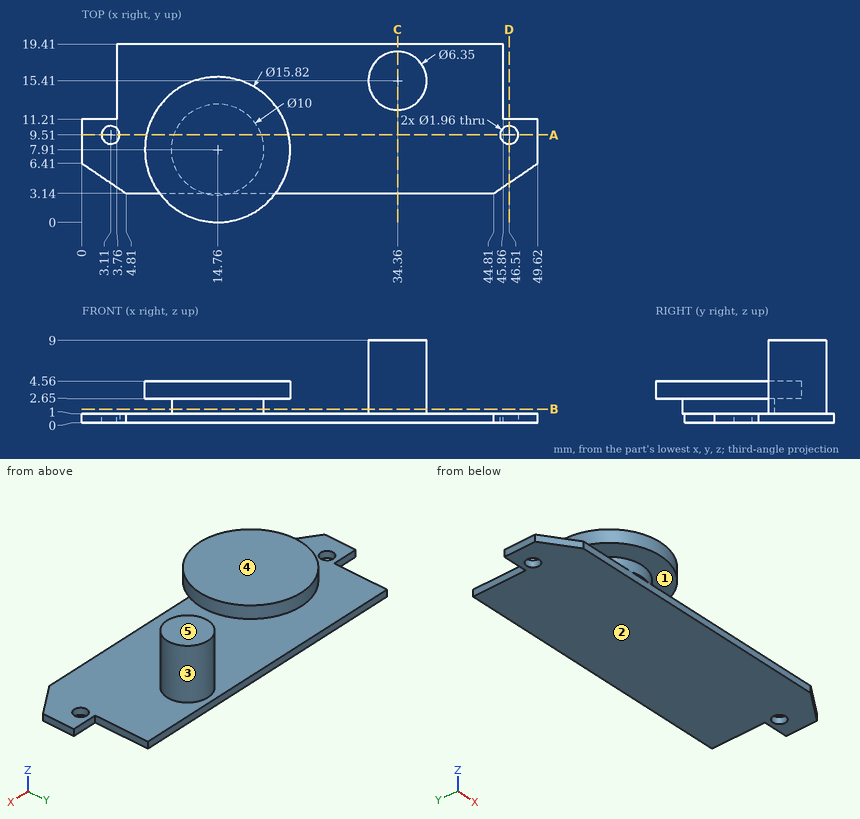
Design review of the part shown in the three views and the two pictorial views. Dimensions are in mm from the part's minimum x, y and z. A direction names the side the tool comes from. Give positions to 0.01 mm unless a question says otherwise; leave off trailing zeros. Write each loop counter-clockwise with the first axis right and the second up, starting at its lowest first coordinate (ties: lowest second). Pieces come first, ordered by that corner, then holes.
(1) Add section D-D (x = 46.51). Give the boundary of the cut face in (y, z).
Checked values:
outline: (4.3, 0) - (8.53, 0) - (8.53, 1) - (4.3, 1) - close; (10.49, 0) - (11.21, 0) - (11.21, 1) - (10.49, 1) - close
(2) Add section B-B (z = 1.5). Give the boundary of the cut face in (x, y) (3 decimals).
Checked values:
outline: circle Ø10 at (14.76, 7.91); circle Ø6.35 at (34.36, 15.41)
(3) Wall thickness on line 1 along Z through (x, y) = (33, 8.5); line 2 along Z through (x, y) = (18, 12.25); line 3 along X through (y, z) = (13.5, 0.5): over which ranges is each line inside the solid? List them lowest first.
Checked values:
line 1: z = 0 to 1
line 2: z = 0 to 1, 2.65 to 4.56
line 3: x = 3.76 to 45.86
(4) Tool access review of the marked faces 4 and 5: name each direction out of +Z, -Z, +X, -X, +Y, -Y from which nothing blocks a thin tool from reaching the whole face with its end or side.
Checked values:
face 4: +Z, -X, +Y, -Y
face 5: +Z, +X, -X, +Y, -Y
(5) Mouldability with a two-part tool opening along Z and no side actions: class the marked faces 1, 2 and 3 as +Z half, -Z half, draft (parallel to the pull), parting line (faces both ways), or undercut.
Checked values:
face 1: undercut
face 2: -Z half
face 3: draft
(6) Add section C-C (x = 34.36). Give the boundary of the cut face in (y, z) (3 decimals).
Checked values:
outline: (3.14, 0) - (19.41, 0) - (19.41, 1) - (18.585, 1) - (18.585, 9) - (12.235, 9) - (12.235, 1) - (3.14, 1) - close
(7) Clearance check with flat-ended pins moving along their axes: pin 1 Ø10 at (x, y) = (17.5, 12.5) entering from +Z; pin 2 Ø1.1 at (y, z) = (14, 0.5) entering from +X; pin 3 Ø0.8 at (y, z) = (13.5, 0.5) entering from -X; pin 4 Ø1.6 at (x, y) = (3.11, 9.51) entering from -Z. State where each tip first meets the part, or that it passes through.
Checked values:
pin 1: stops at z = 4.56
pin 2: stops at x = 45.86
pin 3: stops at x = 3.76
pin 4: passes through
(8) Add section A-A (y = 9.51). Give the boundary of the cut face in (x, z), and give its area (3 significant figures).
Checked values:
outline: (0, 0) - (2.13, 0) - (2.13, 1) - (0, 1) - close; (4.09, 0) - (45.53, 0) - (45.53, 1) - (19.5, 1) - (19.5, 2.65) - (22.51, 2.65) - (22.51, 4.56) - (7.01, 4.56) - (7.01, 2.65) - (10.02, 2.65) - (10.02, 1) - (4.09, 1) - close; (47.49, 0) - (49.62, 0) - (49.62, 1) - (47.49, 1) - close
area: 90.9 mm2
